```python
from build123d import *

# Parameters (mm, degrees)
SKETCH1_W           = 16
SKETCH1_H           = 31
BOSS_EXTRUDE1_DEPTH = 40
SHELL1_T            = -1.5
SKETCH2_W           = 13
SKETCH2_H           = 4
CUT_EXTRUDE1_DEPTH  = 1.5
SKETCH3_W           = 13.5
SKETCH3_H           = 21
CUT_EXTRUDE2_DEPTH  = 1.5


with BuildPart() as part:
    # Sketch1 → Boss-Extrude1 (new body)
    with BuildSketch(Plane(origin=(0, 0, 0), x_dir=(1, 0, 0), z_dir=(0, 1, 0))):
        with Locations((8, -15.5)):
            Rectangle(SKETCH1_W, SKETCH1_H)
    extrude(amount=BOSS_EXTRUDE1_DEPTH)

    # Shell1
    shell1_openings = [part.faces().sort_by_distance(p)[0] for p in [
        (8, 0, 15.5),
    ]]
    offset(amount=SHELL1_T, openings=shell1_openings, kind=Kind.INTERSECTION)

    # Sketch2 → Cut-Extrude1 (cut)
    with BuildSketch(Plane(origin=(0, 40, 0), x_dir=(1, 0, 0), z_dir=(0, 1, 0))):
        with Locations((8, -7)):
            Rectangle(SKETCH2_W, SKETCH2_H)
    extrude(amount=-CUT_EXTRUDE1_DEPTH, mode=Mode.SUBTRACT)

    # Sketch3 → Cut-Extrude2 (cut)
    with BuildSketch(Plane(origin=(0, 0, 0), x_dir=(-1, 0, 0), z_dir=(0, 0, -1))):
        with Locations((-8.031141197, 9.5)):
            Rectangle(SKETCH3_W, SKETCH3_H)
    extrude(amount=-CUT_EXTRUDE2_DEPTH, mode=Mode.SUBTRACT)


solid = part.part
```
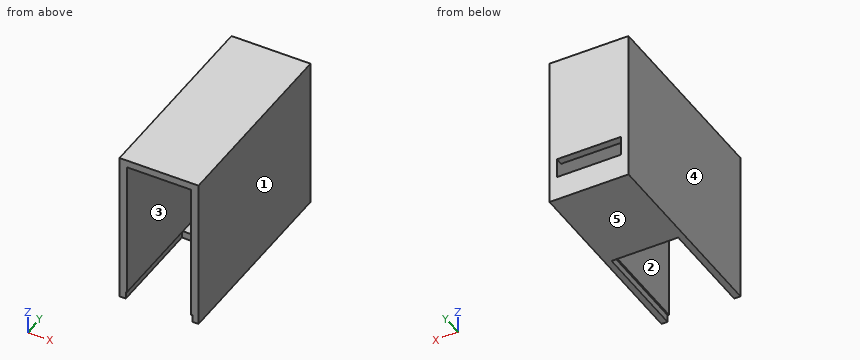
The model under review builds one solid part; all positions refer to its coordinate system, in mm. Face numbers are marked on the shaded views. A direction names the side the tool comes from. Coordinates: 2 decimals unless noted, no trailing zeros. Loops run counter-clockwise (first coordinate to the right, second up) from the corner with the lowest first, then second, coordinate; pieces in that order, holes last. Notation, with made-up numbers: (-39, -15) -> (-28, -15) arc R28 ccw to (-28, 19) -> close; hole circle Ø2 at (-10.75, -20.75). An arc over 180 degrees is marked (long way). Answer as CSV lines item,"result".
Item 1: Draft analysis for pull direction Z (two halves, no side actions). For the marked faces 3, 4 and 5, state which applies: +Z half, -Z half, draft (parallel to the pull), parting line (faces both ways), or undercut.
Results below:
face 3,"undercut"
face 4,"draft"
face 5,"-Z half"
Item 2: For L1, parallel to Z at x = 9.25, y = 24; L2, parallel to X at y = 25, z = 17; L3, parallel to Y at x = 3.25, z = 20.5, list the stretches that pass through material, from the lowest coordinate up.
Results below:
L1,"z = 0 to 1.5, 29.5 to 31"
L2,"x = 0 to 1.5, 14.5 to 16"
L3,"y = 38.5 to 40"
Item 3: Insertion check: pin 1 (1.6 mm diameter, centred on x = 10.5, z = 1, fed in from -Y); pin 2 (1 mm diameter, centred on x = 5.5, z = 4, fed in from -Y); pin 3 (5 mm diameter, centred on y = 34, z = 11, fed in from -X). Each pin has a flat end and moves straight along its axis. Give the tip position at first contact, or say it passes through.
Results below:
pin 1,"stops at y = 20"
pin 2,"stops at y = 38.5"
pin 3,"stops at x = 0"
Item 4: Take a section at B-B, the plane z = 6.5. State the section outline as (x, y) points, and give its area (3 significant figures).
Results below:
outline,"(0, 0) -> (1.5, 0) -> (1.5, 40) -> (0, 40) -> close; (14.5, 0) -> (16, 0) -> (16, 40) -> (14.5, 40) -> close"
area,"120 mm2"
Item 5: Take a section at C-C, the plane y = 21.5. State the section outline as (x, z) points, and give its area (3 significant figures).
Results below:
outline,"(0, 0) -> (16, 0) -> (16, 31) -> (0, 31) -> close; hole (1.5, 1.5) -> (14.5, 1.5) -> (14.5, 29.5) -> (1.5, 29.5) -> close"
area,"132 mm2"
Item 6: Take a section at A-A, the plane x = 8. State the section outline as (y, z) points.
Results below:
outline,"(0, 29.5) -> (38.5, 29.5) -> (38.5, 9) -> (40, 9) -> (40, 31) -> (0, 31) -> close; (20, 0) -> (40, 0) -> (40, 5) -> (38.5, 5) -> (38.5, 1.5) -> (20, 1.5) -> close"
Item 7: Take a section at D-D, the plane z = 10.5. State the section outline as (x, y) points, and give its area (4 significant figures).
Results below:
outline,"(0, 0) -> (1.5, 0) -> (1.5, 38.5) -> (14.5, 38.5) -> (14.5, 0) -> (16, 0) -> (16, 40) -> (0, 40) -> close"
area,"139.5 mm2"
Item 8: Machinability: for the marked faces 1 and 2, which of the approach directions +Z, -Z, +X, -X, +Y, -Y give a long, thin tool a straight path to every point of the face, cutting with its end or side? Answer none if there is none.
Results below:
face 1,"+Z, -Z, +X, +Y, -Y"
face 2,"-Y"
